The model under review builds one solid part; all positions refer to its coordinate system, in mm. A direction names the side the tool comes from. Give positions to 0.01 mm unless a question says otherwise; leave off trailing zeros. Loops run counter-clockwise (first coordinate to the right, second up) from the corner with the lowest first, then second, coordinate; pieces in that order, holes last. Notation, with made-up numbers: M 17.25,47 L 57.25,47 A34 cw 57.25,84 Z; hole C -7,65 d5. An arc over 180 degrees is marked long. Put each result on its own line as item: value. Start each with the question number.
```python
from build123d import *

# Parameters (mm, degrees)
SKETCH1_W           = 15
SKETCH1_H           = 50
BOSS_EXTRUDE1_DEPTH = 40
BOSS_EXTRUDE2_DEPTH = 40
SKETCH1_6_W         = 15
SKETCH1_6_H         = 50
SKETCH1_6_R         = 1.75
BOSS_EXTRUDE3_DEPTH = 12
SKETCH2_W           = 1.4
SKETCH2_H           = 23
CUT_EXTRUDE1_DEPTH  = 30
SKETCH3_W           = 1.4
SKETCH3_H           = 23
CUT_EXTRUDE2_DEPTH  = 30
SKETCH4_R           = 1.75
CUT_EXTRUDE5_DEPTH  = 25
SKETCH5_R           = 4
SKETCH5_R_2         = 1.75
BOSS_EXTRUDE4_DEPTH = 1.5
SKETCH6_R           = 4
SKETCH6_R_2         = 1.75
BOSS_EXTRUDE5_DEPTH = 1.5


with BuildPart() as part:
    # Sketch1 → Boss-Extrude1 (new body)
    with BuildSketch(Plane(origin=(0, 0, 0), x_dir=(1, 0, 0), z_dir=(0, 1, 0))):
        with Locations((-117.5, 0)):
            Rectangle(SKETCH1_W, SKETCH1_H)
    extrude(amount=BOSS_EXTRUDE1_DEPTH)



with BuildPart() as body_2:
    # Sketch1_4 → Boss-Extrude2 (new body)
    with BuildSketch(Plane(origin=(0, 0, 0), x_dir=(1, 0, 0), z_dir=(0, 1, 0))):
        Polygon((125, 25), (110, 25), (110, 0), (110, -25), (125, -25), align=None)
    extrude(amount=BOSS_EXTRUDE2_DEPTH)


with BuildPart() as part_1:
    add(part.part)

    add(body_2.part)  # Boss-Extrude3 merges body 2
    # Sketch1_6 → Boss-Extrude3 (add)
    # profile 1 of 3: a face of its own
    with BuildSketch(Plane(origin=(0, 0, 0), x_dir=(1, 0, 0), z_dir=(0, 1, 0))):
        with Locations((-117.5, 0)):
            Rectangle(SKETCH1_6_W, SKETCH1_6_H)
    # profile 2 of 3: a face of its own
    with BuildSketch(Plane(origin=(0, 0, 0), x_dir=(1, 0, 0), z_dir=(0, 1, 0))):
        Polygon((110, 25), (-110, 25), (-110, -25), (110, -25), (110, 0), align=None)
        with Locations(Location((-51.006782466, -9.590411403, 0), (0, 0, 270))):
            Circle(SKETCH1_6_R, mode=Mode.SUBTRACT)
        with Locations(Location((51.006782466, -9.590411403, 0), (0, 0, 270))):
            Circle(SKETCH1_6_R, mode=Mode.SUBTRACT)
        with Locations(Location((51.006782466, 9.590411403, 0), (0, 0, 270))):
            Circle(SKETCH1_6_R, mode=Mode.SUBTRACT)
    # profile 3 of 3: a face of its own
    with BuildSketch(Plane(origin=(0, 0, 0), x_dir=(1, 0, 0), z_dir=(0, 1, 0))):
        Polygon((125, 25), (110, 25), (110, 0), (110, -25), (125, -25), align=None)
    extrude(amount=BOSS_EXTRUDE3_DEPTH)

    # Sketch2 → Cut-Extrude1 (cut)
    with BuildSketch(Plane(origin=(0, 40, 0), x_dir=(1, 0, 0), z_dir=(0, 1, 0))):
        with Locations((-117.45, 0)):
            Rectangle(SKETCH2_W, SKETCH2_H)
    extrude(amount=-CUT_EXTRUDE1_DEPTH, mode=Mode.SUBTRACT)

    # Sketch3 → Cut-Extrude2 (cut)
    with BuildSketch(Plane(origin=(0, 40, 0), x_dir=(1, 0, 0), z_dir=(0, 1, 0))):
        with Locations((117.5, 0)):
            Rectangle(SKETCH3_W, SKETCH3_H)
    extrude(amount=-CUT_EXTRUDE2_DEPTH, mode=Mode.SUBTRACT)

    # Sketch4 → Cut-Extrude5 (cut)
    with BuildSketch(Plane(origin=(0, 12, 0), x_dir=(1, 0, 0), z_dir=(0, 1, 0))):
        with Locations(Location((-51.006782466, 9.590411403, 0), (0, 0, 270))):
            Circle(SKETCH4_R)
    extrude(amount=-CUT_EXTRUDE5_DEPTH, mode=Mode.SUBTRACT)

    # Sketch5 → Boss-Extrude4 (add)
    with BuildSketch(Plane(origin=(0, 12, 0), x_dir=(1, 0, 0), z_dir=(0, 1, 0))):
        with Locations(Location((-51.006782466, -9.590411403, 0), (0, 0, 270))):
            Circle(SKETCH5_R)
        with Locations(Location((-51.006782466, -9.590411403, 0), (0, 0, 270))):
            Circle(SKETCH5_R_2, mode=Mode.SUBTRACT)
    extrude(amount=BOSS_EXTRUDE4_DEPTH)

    # Sketch6 → Boss-Extrude5 (add)
    # profile 1 of 3: a face of its own
    with BuildSketch(Plane(origin=(0, 12, 0), x_dir=(1, 0, 0), z_dir=(0, 1, 0))):
        with Locations(Location((-51.006782466, 9.590411403, 0), (0, 0, 270))):
            Circle(SKETCH6_R)
        with Locations(Location((-51.006782466, 9.590411403, 0), (0, 0, 270))):
            Circle(SKETCH6_R_2, mode=Mode.SUBTRACT)
    # profile 2 of 3: a face of its own
    with BuildSketch(Plane(origin=(0, 12, 0), x_dir=(1, 0, 0), z_dir=(0, 1, 0))):
        with Locations(Location((51.006782466, 9.590411403, 0), (0, 0, 270))):
            Circle(SKETCH6_R)
        with Locations(Location((51.006782466, 9.590411403, 0), (0, 0, 270))):
            Circle(SKETCH6_R_2, mode=Mode.SUBTRACT)
    # profile 3 of 3: a face of its own
    with BuildSketch(Plane(origin=(0, 12, 0), x_dir=(1, 0, 0), z_dir=(0, 1, 0))):
        with Locations(Location((51.006782466, -9.590411403, 0), (0, 0, 270))):
            Circle(SKETCH6_R)
        with Locations(Location((51.006782466, -9.590411403, 0), (0, 0, 270))):
            Circle(SKETCH6_R_2, mode=Mode.SUBTRACT)
    extrude(amount=BOSS_EXTRUDE5_DEPTH)


solid = part_1.part
```
Item 1: Consider section C-C, the plane x = 10.5. Write out the cut boundary in (y, z), plus the area to 3 significant figures.
Item 2: To check wall thickness, follow L1, parallel to X at y = 21.5, z = 6.5; L2, parallel to X at y = 17.5, z = -12.5; L3, parallel to X at y = 6, z = -11. State the ranges of each line that lie inside material, in increasing order. Write a range as [from, to].
Item 3: Consider section A-A, the plane y = 18.5. Write out the cut boundary in (x, z), plus the area to 3 significant figures.
Item 4: Draft analysis for pull direction Z (two halves, no side actions). For faces 1 (the cylindrical face through (-54.9, 12.7, -10.5)), 2 (the flat face through (-30, 11, -25)), 3 (the flat face through (-2, 0, 0)), state which applies: +Z half, -Z half, draft (parallel to the pull), parting line (faces both ways), or undercut.
Item 5: Consider section B-B, the plane z = -1. Write out the cut boundary in (x, y).
Item 6: Clearance check with flat-ended pins moving along their axes: pin 1 Ø3 at (x, z) = (-40, 11.5) entering from +Y; pin 2 Ø4 at (x, z) = (-50.5, -8) entering from +Y; pin 3 Ø0.7 at (x, z) = (-117.5, -5) entering from +Y. State where each tip first meets the part, or that it passes through.
Item 7: Tool access review of faces 4 (the flat face through (119, 40, 0)), 5 (the cylindrical face through (47.102, 12.74, -10.458)), 6 (the flat face through (-53, 13.5, 10)): name each direction out of +Z, -Z, +X, -X, +Y, -Y from which nothing blocks a thin tool from reaching the whole face with its end or side.
Report:
1. outline: M 0,-25 L 12,-25 L 12,25 L 0,25 Z
1. area: 600 mm²
2. L1: [-125, -118.15], [-116.75, -110], [110, 116.8], [118.2, 125]
2. L2: [-125, -110], [110, 125]
2. L3: [-125, -52.04], [-49.97, 49.97], [52.04, 125]
3. outline: M -125,-25 L -110,-25 L -110,25 L -125,25 Z; M 110,-25 L 125,-25 L 125,25 L 110,25 Z; hole M -118.15,-11.5 L -116.75,-11.5 L -116.75,11.5 L -118.15,11.5 Z; hole M 116.8,-11.5 L 118.2,-11.5 L 118.2,11.5 L 116.8,11.5 Z
3. area: 1,440 mm²
4. face 1: undercut
4. face 2: -Z half
4. face 3: draft
5. outline: M -125,0 L 125,0 L 125,40 L 118.2,40 L 118.2,10 L 116.8,10 L 116.8,40 L 110,40 L 110,12 L -110,12 L -110,40 L -116.75,40 L -116.75,10 L -118.15,10 L -118.15,40 L -125,40 Z
6. pin 1: y = 12
6. pin 2: y = 13.5
6. pin 3: y = 10
7. face 4: +Z, -Z, +X, -X, +Y
7. face 5: +Y
7. face 6: +Z, -Z, +Y
